Can you work these out from the model? Positions are in its coordinate system, mm. A direction names the side the tool comes from. Coordinates: 2 decimals unless noted, no trailing zeros. Loops run counter-clockwise (first coordinate to the right, second up) from the corner with the lowest first, then second, coordinate; pieces in that order, holes last. Notation, with made-up numbers: M 75,-37.5 L 102,-37.5 A27 cw 102,-3.5 Z; hole C -10,39.25 d1. An arc over 180 degrees is marked long. Return JSON: item names as keys, results as strings. Group by question number.
```python
from build123d import *

# Parameters (mm, degrees)
F1_DEPTH = 17
F4_DEPTH = 13
F6_DEPTH = 2.001
F8_DEPTH = 2.001


with BuildPart() as f1:
    # F0 (on Front) → F1 (new body)
    with BuildSketch(Plane.XZ):
        Polygon((0, 20), (0, 0), (20, 0), (18, 2), (2, 2), (2, 18), align=None)
        Polygon((18, 2), (2, 18), (2, 2), align=None)
    extrude(amount=-F1_DEPTH)

    # F3 (on offset) → F4 (cut)
    with BuildSketch(Plane.XZ.offset(-2)):
        Polygon((2, 2), (18, 2), (2, 18), align=None)
    extrude(amount=-F4_DEPTH, mode=Mode.SUBTRACT)

    # F5 (on face) → F6 (cut, through all)
    with BuildSketch(Plane.YZ.offset(2)):
        with BuildLine():
            ThreePointArc((11.5, 12), (8.5, 15), (5.5, 12))
            Line((5.5, 12), (5.5, 8))
            ThreePointArc((5.5, 8), (8.5, 5), (11.5, 8))
            Line((11.5, 8), (11.5, 12))
        make_face()
    extrude(amount=-F6_DEPTH, mode=Mode.SUBTRACT)

    # F7 (on face) → F8 (cut, through all)
    with BuildSketch(Plane.XY.offset(2)):
        with BuildLine():
            ThreePointArc((8, 11.5), (5, 8.5), (8, 5.5))
            Line((8, 5.5), (12, 5.5))
            ThreePointArc((12, 5.5), (15, 8.5), (12, 11.5))
            Line((12, 11.5), (8, 11.5))
        make_face()
    extrude(amount=-F8_DEPTH, mode=Mode.SUBTRACT)


solid = f1.part
```
1) For pin 1 (3 mm diameter, centred on x = 9, y = 15.5, fed in from +Z); pin 2 (6 mm diameter, centred on x = 7, y = 10.5, fed in from +Z); pin 3 (4 mm diameter, centred on y = 4.5, z = 10.5, fed in from +X), each with a flat end and sliding along its axis, tell me the tip position at first contact or that it passes through.
2) Suppose I cut it at B-B, the plane z = 8.5. List the corners of the cut face in (x, y) for me.
3) Suppose I cut it at D-D, the plane z = 15.75. List the corners of the cut face in (x, y) for me, then the cut area to 3 significant figures.
4) Suppose I cut it at C-C, the plane x = 11.5. List the corners of the cut face in (y, z) for me.
5) If I drill on line 1 (Y direction, x = 5, z = 12); line 2 (Z direction, x = 13, y = 5), over which ranges is the centre line in solid material (lowest first)? Write a range as from..to.
6) If we mould it in two halves opening along X, with no side actions, what happens to faces 1 (the face through (10, 1, 10)), 2 (the face through (5, 17, 6)), 3 (the face through (0, 5, 10)), 4 (the face through (5, 8.6, 1))? For each: +X half, -X half, draft (parallel to the pull), parting line (faces both ways), or undercut.
7) Suppose I cut it at A-A, the plane y = 8.5. List the corners of the cut face in (x, z) for me, then the cut area to 3 significant figures.
8) For faces 5 (the face through (15, 8.4, 1)), 6 (the face through (6, 2, 7)), 7 (the face through (1, 5.5, 10)), 8 (the face through (10, 5, 0)), which set-ups out of +Z, -Z, +X, -X, +Y, -Y let a thin tool reach every point of the face, with its end or its side?
Returned:
{
 "1": {"pin 1": "stops at z = 12.5", "pin 2": "stops at z = 2", "pin 3": "stops at x = 2"},
 "2": {"outline": "M 0,0 L 11.5,0 L 11.5,2 L 2,2 L 2,5.5 L 0,5.5 Z; M 0,11.5 L 2,11.5 L 2,15 L 11.5,15 L 11.5,17 L 0,17 Z"},
 "3": {"outline": "M 0,0 L 4.25,0 L 4.25,2 L 2,2 L 2,15 L 4.25,15 L 4.25,17 L 0,17 Z", "area": "43.0 mm²"},
 "4": {"outline": "M 0,0 L 5.5,0 L 5.5,2 L 2,2 L 2,8.5 L 0,8.5 Z; M 11.5,0 L 17,0 L 17,8.5 L 15,8.5 L 15,2 L 11.5,2 Z"},
 "5": {"line 1": "y = 0..2, 15..17", "line 2": "z = 0..2"},
 "6": {"face 1": "+X half", "face 2": "draft", "face 3": "-X half", "face 4": "undercut"},
 "7": {"outline": "M 0,0 L 5,0 L 5,2 L 2,2 L 2,5 L 0,5 Z; M 0,15 L 2,15 L 2,18 L 0,20 Z; M 15,0 L 20,0 L 18,2 L 15,2 Z", "area": "32.0 mm²"},
 "8": {"face 5": "+Z, -Z", "face 6": "+Z, +X", "face 7": "+X, -X", "face 8": "-Z, +X, -X, +Y, -Y"}
}
